Geometry check sheet. Reference: the model listing, model coordinates, mm. A direction names the side the tool comes from. Give positions to 0.01 mm unless a question says otherwise; leave off trailing zeros. Loops run counter-clockwise (first coordinate to the right, second up) from the corner with the lowest first, then second, coordinate; pieces in that order, holes last. Notation, with made-up numbers: (-16, -36.5) - (23, -36.5) arc R29 ccw to (23, -15.5) - close; hole circle Ø6 at (-20, -37). An arc over 180 degrees is marked (long way). One line per question, with ' | ' between items. Start each with the question number.
from build123d import *

# Parameters (mm, degrees)
SKETCH1_W           = 63.5
SKETCH1_H           = 25.4
SKETCH1_W_2         = 3.175
SKETCH1_H_2         = 11.1125
BOSS_EXTRUDE1_DEPTH = 3.175
SKETCH2_W           = 53.975
SKETCH2_H           = 9.525
CUT_EXTRUDE1_DEPTH  = 72.419858933


with BuildPart() as part:
    # Sketch1 → Boss-Extrude1 (new body)
    with BuildSketch(Plane(origin=(0, 0, 0), x_dir=(1, 0, 0), z_dir=(0, 1, 0))):
        with Locations((31.75, 12.7)):
            Rectangle(SKETCH1_W, SKETCH1_H)
        with Locations((-1.5875, 19.84375)):
            Rectangle(SKETCH1_W_2, SKETCH1_H_2)
        with Locations((-1.5875, 5.55625)):
            Rectangle(SKETCH1_W_2, SKETCH1_H_2)
        with Locations((65.0875, 19.84375)):
            Rectangle(SKETCH1_W_2, SKETCH1_H_2)
        with Locations((65.0875, 5.55625)):
            Rectangle(SKETCH1_W_2, SKETCH1_H_2)
    extrude(amount=BOSS_EXTRUDE1_DEPTH)

    # Sketch2 → Cut-Extrude1 (cut, through all)
    with BuildSketch(Plane(origin=(0, 3.175, 0), x_dir=(1, 0, 0), z_dir=(0, 1, 0))):
        with Locations((31.75, 12.7)):
            Rectangle(SKETCH2_W, SKETCH2_H)
    extrude(amount=-CUT_EXTRUDE1_DEPTH, mode=Mode.SUBTRACT)


solid = part.part
(1) Depth check by flat-ended pin: pin 1 Ø1 at (y, z) = (1, -12.5) entering from +X; pin 2 Ø1 at (y, z) = (1, -12.5) entering from -X. Enter the tip coordinate at first touch or a pass-through.
(2) Tool access check on faces 4 (the face through (66.675, 2, -20)), 5 (the face through (58.738, 2, -13)), 6 (the face through (-2, 2, -11.112)), 7 (the face through (63.5, 2, -13)). Record the directions out of +Z, -Z, +X, -X, +Y, -Y that give a thin tool (end or side, any length) a straight path to the whole face; none if there is none.
(3) Section check B-B, the plane y = 0.5. Record the boundary of the cut face in (x, z) (1 decimal), and give its area (3 significant figures).
(4) Mould release check, pull along X, two halves, no side actions. Record for faces 1 (the face through (-3.175, 2, -5)), 2 (the face through (31, 2, -17.462)), 3 (the face through (-2, 2, -14.288)): pulls with the +X half, pulls with the -X half, needs draft (parallel to the pull), parting line crosses it, or undercut.
(5) Section check C-C, the plane x = 55.5. Record the boundary of the cut face in (y, z) (1 decimal).
(6) Section check A-A, the plane z = -15. Record the boundary of the cut face in (x, y) (1 decimal), and give its area (3 significant figures).
(7) Material ranges on line 1 (Z direction, x = 6.5, y = 1.4); line 2 (X direction, y = 1.05, z = -13); line 3 (X direction, y = 1.85, z = -17) (1 decimal), recorded low to high.
Numbers:
1) pin 1: x = 63.5 | pin 2: x = 0
2) face 4: +Z, -Z, +X, +Y, -Y | face 5: +Y, -Y | face 6: -X, +Y, -Y | face 7: +X, +Y, -Y
3) outline: (-3.2, -25.4) - (66.7, -25.4) - (66.7, -14.3) - (63.5, -14.3) - (63.5, -11.1) - (66.7, -11.1) - (66.7, 0) - (-3.2, 0) - (-3.2, -11.1) - (0, -11.1) - (0, -14.3) - (-3.2, -14.3) - close; hole (4.8, -17.5) - (58.7, -17.5) - (58.7, -7.9) - (4.8, -7.9) - close | area: 1,240 mm^2
4) face 1: pulls with the -X half | face 2: undercut | face 3: needs draft
5) outline: (0, -25.4) - (3.2, -25.4) - (3.2, -17.5) - (0, -17.5) - close; (0, -7.9) - (3.2, -7.9) - (3.2, 0) - (0, 0) - close
6) outline: (-3.2, 0) - (4.8, 0) - (4.8, 3.2) - (-3.2, 3.2) - close; (58.7, 0) - (66.7, 0) - (66.7, 3.2) - (58.7, 3.2) - close | area: 50.4 mm^2
7) line 1: -25.4 to -17.46, -7.94 to 0 | line 2: 0 to 4.76, 58.74 to 63.5 | line 3: -3.2 to 4.8, 58.7 to 66.7
